from build123d import *

# Parameters (mm, degrees)
EXTRUDE_1_DEPTH     = 30
SKETCH_2_R          = 0.64072886
CUT_EXTRUDE_2_DEPTH = 7


with BuildPart() as part:
    # 草图1 → 凸台-拉伸1 (new body)
    with BuildSketch(Plane.XY):
        Polygon((28.041755138, 1.822698956), (-1.958244862, 1.822698956), (-1.958244862, -28.177301044), (0, -28), (1, -27.237055845), (0, -27.237055845), (0, 0), (27.305301665, 0), (27.305301665, -1), (28, 0), align=None)
    extrude(amount=EXTRUDE_1_DEPTH)

    # 草图2 → 切除-拉伸2 (cut)
    with BuildSketch(Plane(origin=(0, 0, 0), x_dir=(1, 0, 0), z_dir=(0, 1, 0))):
        with Locations((2.910195006, -3.432793696)):
            Circle(SKETCH_2_R)
        with Locations((2.910195006, -25.623781676)):
            Circle(SKETCH_2_R)
        with Locations((22.147853718, -3.432793696)):
            Circle(SKETCH_2_R)
        with Locations((22.147853718, -25.623781676)):
            Circle(SKETCH_2_R)
    extrude(amount=CUT_EXTRUDE_2_DEPTH, mode=Mode.SUBTRACT)


solid = part.part
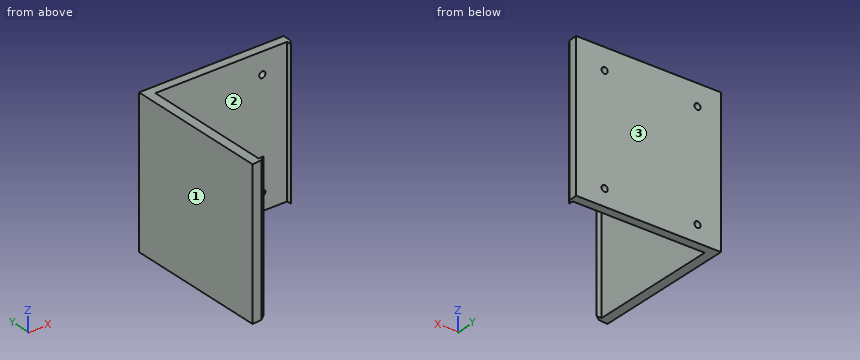
Design review of the part built by this model. Coordinates are the model's own, in mm. Face numbers are marked on the shaded views. Round coordinates to 2 decimals unless told otherwise and drop trailing zeros. Order: outer loops, then holes, each group sorted by start corner. A loop starts at its lowest first (then second) coordinate and runs counter-clockwise, first axis right, second up. Notation, with made-up numbers: M 33.25,43.25 L 77.25,43.25 A12 ccw 77.25,62.25 Z; hole C -34,7 d8. An arc over 180 degrees is marked long. Answer as CSV lines item,"result". Start each with the question number.
1) Add section B-B (x = 24). Give the boundary of the cut face in (y, z), then the cut area to 3 significant figures.
2) Add section A-A (z = 19). Give the boundary of the cut face in (x, y), then the cut area to 3 significant figures.
3) For pin 1 Ø6 at (y, z) = (-21.5, 9) entering from +X; pin 2 Ø13.5 at (x, z) = (11, 22) entering from -Y, all flat-tipped, find the tip position at first contact; note any pin that passes through.
4) Add section C-C (y = -11). Give the boundary of the cut face in (x, z).
5) Wall thickness on line 1 along X through (y, z) = (-19.25, 17); line 2 along Y through (x, z) = (23, 9.5); line 3 along Y through (x, z) = (-0.25, 15): over which ranges is each line inside the solid? List them lowest first. Write a range as [from, to].
6) The part is to be moulded in two halves that separate along X. For the marked faces 1, 2 and 3, say which applies: +X half, -X half, draft (parallel to the pull), parting line (faces both ways), or undercut.
Resolved:
1,outline,"M 0,0 L 1.82,0 L 1.82,30 L 0,30 Z"
1,area,"54.7 mm^2"
2,outline,"M -1.96,-28.18 L 0,-28 L 1,-27.24 L 0,-27.24 L 0,0 L 27.31,0 L 27.31,-1 L 28,0 L 28.04,1.82 L -1.96,1.82 Z"
2,area,"110 mm^2"
3,pin 1,"x = 0"
3,pin 2,"y = 0"
4,outline,"M -1.96,0 L 0,0 L 0,30 L -1.96,30 Z"
5,line 1,"[-1.96, 0]"
5,line 2,"[0, 1.82]"
5,line 3,"[-28.02, 1.82]"
6,face 1,"-X half"
6,face 2,"undercut"
6,face 3,"draft"
